Source: CAD feature listing. Evaluate the final solid. Frame: model axes, mm. A direction names the side the tool comes from. Round coordinates to 2 decimals unless told otherwise and drop trailing zeros. Answer in a Markdown table with one row per item. Add a question column.
Item 1: Mould query, pull axis Y, two halves, no side actions, for faces 1 (the face through (-2, 212.5, 7)), 2 (the face through (16, 158, 6)), 3 (the face through (-161, -3, 7)). Classes: released by +Y, released by -Y, zero draft, split by the parting line, or undercut.
Item 2: Set-up query: faces 4 (the face through (134, -112, 8)), 5 (the face through (-2, 3, 0)). Return all of +Z, -Z, +X, -X, +Y, -Y with unobstructed straight access to the full face (end or side cutting, diameter ignored); none if empty.
Item 3: Material intervals for probe 1 along Y at (x, z) = (-14.3, 1.5); probe 2 along Y at (x, z) = (152.5, 6.5); probe 3 along X at (y, z) = (144.5, 4), sorted ascending.
Item 4: Contact query for flat-ended pins moving along their axis: pin 1 (3.5 mm diameter, centred on x = 96.5, y = 109.5, fed in from +Z); pin 2 (3 mm diameter, centred on x = -94.5, y = -111.5, fed in from +Z). Output: stop coordinate, or through.
from build123d import *

# Parameters (mm, degrees)
SZKIC1_W                       = 322
SZKIC1_H                       = 425
DODANIE_WYCI_GNI_CIE1_DEPTH    = 15
SZKIC2_R                       = 3
WYTNIJ_WYCI_GNI_CIE1_DEPTH     = 15
SZKIC3_R                       = 5
WYTNIJ_WYCI_GNI_CIE2_DEPTH     = 7
SZYK_LINIOWY1_COUNT            = 2
SZYK_LINIOWY1_PITCH            = 35
SZYK_LINIOWY1_COUNT_DIR2       = 2
SZYK_LINIOWY1_PITCH_DIR2       = 35
SZYK_LINIOWY2_COUNT            = 2
SZYK_LINIOWY2_PITCH            = 228
SZYK_LINIOWY2_COUNT_DIR2       = 2
SZYK_LINIOWY2_PITCH_DIR2       = 254
SZYK_LINIOWY2_COPY_1_SKETCH_R  = 3
SZYK_LINIOWY2_COPY_1_DEPTH     = 15
SZYK_LINIOWY2_COPY_2_SKETCH_R  = 3
SZYK_LINIOWY2_COPY_2_DEPTH     = 15
SZYK_LINIOWY2_COPY_3_SKETCH_R  = 3
SZYK_LINIOWY2_COPY_3_DEPTH     = 15
SZYK_LINIOWY2_COPY_4_SKETCH_R  = 3
SZYK_LINIOWY2_COPY_4_DEPTH     = 15
SZYK_LINIOWY2_COPY_5_SKETCH_R  = 3
SZYK_LINIOWY2_COPY_5_DEPTH     = 15
SZYK_LINIOWY2_COPY_6_SKETCH_R  = 3
SZYK_LINIOWY2_COPY_6_DEPTH     = 15
SZYK_LINIOWY2_COPY_7_SKETCH_R  = 3
SZYK_LINIOWY2_COPY_7_DEPTH     = 15
SZYK_LINIOWY2_COPY_8_SKETCH_R  = 3
SZYK_LINIOWY2_COPY_8_DEPTH     = 15
SZYK_LINIOWY2_COPY_9_SKETCH_R  = 3
SZYK_LINIOWY2_COPY_9_DEPTH     = 15
SZYK_LINIOWY2_COPY_10_SKETCH_R = 5
SZYK_LINIOWY2_COPY_10_DEPTH    = 7
SZYK_LINIOWY2_COPY_11_SKETCH_R = 5
SZYK_LINIOWY2_COPY_11_DEPTH    = 7
SZYK_LINIOWY2_COPY_12_SKETCH_R = 5
SZYK_LINIOWY2_COPY_12_DEPTH    = 7
SZYK_LINIOWY2_COPY_13_SKETCH_R = 5
SZYK_LINIOWY2_COPY_13_DEPTH    = 7
SZYK_LINIOWY2_COPY_14_SKETCH_R = 5
SZYK_LINIOWY2_COPY_14_DEPTH    = 7
SZYK_LINIOWY2_COPY_15_SKETCH_R = 5
SZYK_LINIOWY2_COPY_15_DEPTH    = 7
SZYK_LINIOWY2_COPY_16_SKETCH_R = 5
SZYK_LINIOWY2_COPY_16_DEPTH    = 7
SZYK_LINIOWY2_COPY_17_SKETCH_R = 5
SZYK_LINIOWY2_COPY_17_DEPTH    = 7
SZYK_LINIOWY2_COPY_18_SKETCH_R = 5
SZYK_LINIOWY2_COPY_18_DEPTH    = 7
SZKIC6_R                       = 4
WYTNIJ_WYCI_GNI_CIE3_DEPTH     = 20
SZKIC7_R                       = 4
WYTNIJ_WYCI_GNI_CIE4_DEPTH     = 20
SZKIC10_R                      = 4
WYTNIJ_WYCI_GNI_CIE5_DEPTH     = 21
SZKIC11_R                      = 4
WYTNIJ_WYCI_GNI_CIE6_DEPTH     = 21
SZKIC12_R                      = 3.999999999
WYTNIJ_WYCI_GNI_CIE7_DEPTH     = 15
SZKIC13_R                      = 6.499999999
WYTNIJ_WYCI_GNI_CIE8_DEPTH     = 9
SZKIC14_R                      = 4
WYTNIJ_WYCI_GNI_CIE9_DEPTH     = 15
SZYK_LINIOWY3_COUNT            = 4
SZYK_LINIOWY3_PITCH            = 133


with BuildPart() as part:
    # Szkic1 → Dodanie-wyciągnięcie1 (new body)
    with BuildSketch(Plane.XY):
        Rectangle(SZKIC1_W, SZKIC1_H)
    extrude(amount=DODANIE_WYCI_GNI_CIE1_DEPTH)

    # Szkic2 → Wytnij-wyciągnięcie1 (cut)
    with BuildSketch(Plane.XY.offset(15)):
        with Locations((-131.5, 144.5)):
            Circle(SZKIC2_R)
    wytnij_wyci_gni_cie1 = extrude(amount=-WYTNIJ_WYCI_GNI_CIE1_DEPTH, mode=Mode.SUBTRACT)

    # Szkic3 → Wytnij-wyciągnięcie2 (cut)
    with BuildSketch(Plane.XY.offset(15)):
        with Locations((-131.5, 144.5)):
            Circle(SZKIC3_R)
    wytnij_wyci_gni_cie2 = extrude(amount=-WYTNIJ_WYCI_GNI_CIE2_DEPTH, mode=Mode.SUBTRACT)

    # Szyk liniowy1: Wytnij-wyciągnięcie1, Wytnij-wyci_gni_cie2 2 × 2
    with Locations(*[(i * SZYK_LINIOWY1_PITCH, -j * SZYK_LINIOWY1_PITCH_DIR2, 0) for i in range(SZYK_LINIOWY1_COUNT) for j in range(SZYK_LINIOWY1_COUNT_DIR2) if (i, j) != (0, 0)]):
        add(wytnij_wyci_gni_cie1, mode=Mode.SUBTRACT)
        add(wytnij_wyci_gni_cie2, mode=Mode.SUBTRACT)

    # Szyk liniowy2: Wytnij-wyciągnięcie1, Wytnij-wyci_gni_cie2 2 × 2
    with Locations(*[(i * SZYK_LINIOWY2_PITCH, -j * SZYK_LINIOWY2_PITCH_DIR2, 0) for i in range(SZYK_LINIOWY2_COUNT) for j in range(SZYK_LINIOWY2_COUNT_DIR2) if (i, j) != (0, 0)]):
        add(wytnij_wyci_gni_cie1, mode=Mode.SUBTRACT)
        add(wytnij_wyci_gni_cie2, mode=Mode.SUBTRACT)

    # Szyk liniowy2 copy 1 sketch → Szyk liniowy2 copy 1 (cut)
    with BuildSketch(Plane(origin=(0, -289, 15), x_dir=(1, 0, 0), z_dir=(0, 0, 1))):
        with Locations((-131.5, 144.5)):
            Circle(SZYK_LINIOWY2_COPY_1_SKETCH_R)
    extrude(amount=-SZYK_LINIOWY2_COPY_1_DEPTH, mode=Mode.SUBTRACT)

    # Szyk liniowy2 copy 2 sketch → Szyk liniowy2 copy 2 (cut)
    with BuildSketch(Plane(origin=(228, -35, 15), x_dir=(1, 0, 0), z_dir=(0, 0, 1))):
        with Locations((-131.5, 144.5)):
            Circle(SZYK_LINIOWY2_COPY_2_SKETCH_R)
    extrude(amount=-SZYK_LINIOWY2_COPY_2_DEPTH, mode=Mode.SUBTRACT)

    # Szyk liniowy2 copy 3 sketch → Szyk liniowy2 copy 3 (cut)
    with BuildSketch(Plane(origin=(228, -289, 15), x_dir=(1, 0, 0), z_dir=(0, 0, 1))):
        with Locations((-131.5, 144.5)):
            Circle(SZYK_LINIOWY2_COPY_3_SKETCH_R)
    extrude(amount=-SZYK_LINIOWY2_COPY_3_DEPTH, mode=Mode.SUBTRACT)

    # Szyk liniowy2 copy 4 sketch → Szyk liniowy2 copy 4 (cut)
    with BuildSketch(Plane(origin=(35, -254, 15), x_dir=(1, 0, 0), z_dir=(0, 0, 1))):
        with Locations((-131.5, 144.5)):
            Circle(SZYK_LINIOWY2_COPY_4_SKETCH_R)
    extrude(amount=-SZYK_LINIOWY2_COPY_4_DEPTH, mode=Mode.SUBTRACT)

    # Szyk liniowy2 copy 5 sketch → Szyk liniowy2 copy 5 (cut)
    with BuildSketch(Plane(origin=(263, 0, 15), x_dir=(1, 0, 0), z_dir=(0, 0, 1))):
        with Locations((-131.5, 144.5)):
            Circle(SZYK_LINIOWY2_COPY_5_SKETCH_R)
    extrude(amount=-SZYK_LINIOWY2_COPY_5_DEPTH, mode=Mode.SUBTRACT)

    # Szyk liniowy2 copy 6 sketch → Szyk liniowy2 copy 6 (cut)
    with BuildSketch(Plane(origin=(263, -254, 15), x_dir=(1, 0, 0), z_dir=(0, 0, 1))):
        with Locations((-131.5, 144.5)):
            Circle(SZYK_LINIOWY2_COPY_6_SKETCH_R)
    extrude(amount=-SZYK_LINIOWY2_COPY_6_DEPTH, mode=Mode.SUBTRACT)

    # Szyk liniowy2 copy 7 sketch → Szyk liniowy2 copy 7 (cut)
    with BuildSketch(Plane(origin=(35, -289, 15), x_dir=(1, 0, 0), z_dir=(0, 0, 1))):
        with Locations((-131.5, 144.5)):
            Circle(SZYK_LINIOWY2_COPY_7_SKETCH_R)
    extrude(amount=-SZYK_LINIOWY2_COPY_7_DEPTH, mode=Mode.SUBTRACT)

    # Szyk liniowy2 copy 8 sketch → Szyk liniowy2 copy 8 (cut)
    with BuildSketch(Plane(origin=(263, -35, 15), x_dir=(1, 0, 0), z_dir=(0, 0, 1))):
        with Locations((-131.5, 144.5)):
            Circle(SZYK_LINIOWY2_COPY_8_SKETCH_R)
    extrude(amount=-SZYK_LINIOWY2_COPY_8_DEPTH, mode=Mode.SUBTRACT)

    # Szyk liniowy2 copy 9 sketch → Szyk liniowy2 copy 9 (cut)
    with BuildSketch(Plane(origin=(263, -289, 15), x_dir=(1, 0, 0), z_dir=(0, 0, 1))):
        with Locations((-131.5, 144.5)):
            Circle(SZYK_LINIOWY2_COPY_9_SKETCH_R)
    extrude(amount=-SZYK_LINIOWY2_COPY_9_DEPTH, mode=Mode.SUBTRACT)

    # Szyk liniowy2 copy 10 sketch → Szyk liniowy2 copy 10 (cut)
    with BuildSketch(Plane(origin=(0, -289, 15), x_dir=(1, 0, 0), z_dir=(0, 0, 1))):
        with Locations((-131.5, 144.5)):
            Circle(SZYK_LINIOWY2_COPY_10_SKETCH_R)
    extrude(amount=-SZYK_LINIOWY2_COPY_10_DEPTH, mode=Mode.SUBTRACT)

    # Szyk liniowy2 copy 11 sketch → Szyk liniowy2 copy 11 (cut)
    with BuildSketch(Plane(origin=(228, -35, 15), x_dir=(1, 0, 0), z_dir=(0, 0, 1))):
        with Locations((-131.5, 144.5)):
            Circle(SZYK_LINIOWY2_COPY_11_SKETCH_R)
    extrude(amount=-SZYK_LINIOWY2_COPY_11_DEPTH, mode=Mode.SUBTRACT)

    # Szyk liniowy2 copy 12 sketch → Szyk liniowy2 copy 12 (cut)
    with BuildSketch(Plane(origin=(228, -289, 15), x_dir=(1, 0, 0), z_dir=(0, 0, 1))):
        with Locations((-131.5, 144.5)):
            Circle(SZYK_LINIOWY2_COPY_12_SKETCH_R)
    extrude(amount=-SZYK_LINIOWY2_COPY_12_DEPTH, mode=Mode.SUBTRACT)

    # Szyk liniowy2 copy 13 sketch → Szyk liniowy2 copy 13 (cut)
    with BuildSketch(Plane(origin=(35, -254, 15), x_dir=(1, 0, 0), z_dir=(0, 0, 1))):
        with Locations((-131.5, 144.5)):
            Circle(SZYK_LINIOWY2_COPY_13_SKETCH_R)
    extrude(amount=-SZYK_LINIOWY2_COPY_13_DEPTH, mode=Mode.SUBTRACT)

    # Szyk liniowy2 copy 14 sketch → Szyk liniowy2 copy 14 (cut)
    with BuildSketch(Plane(origin=(263, 0, 15), x_dir=(1, 0, 0), z_dir=(0, 0, 1))):
        with Locations((-131.5, 144.5)):
            Circle(SZYK_LINIOWY2_COPY_14_SKETCH_R)
    extrude(amount=-SZYK_LINIOWY2_COPY_14_DEPTH, mode=Mode.SUBTRACT)

    # Szyk liniowy2 copy 15 sketch → Szyk liniowy2 copy 15 (cut)
    with BuildSketch(Plane(origin=(263, -254, 15), x_dir=(1, 0, 0), z_dir=(0, 0, 1))):
        with Locations((-131.5, 144.5)):
            Circle(SZYK_LINIOWY2_COPY_15_SKETCH_R)
    extrude(amount=-SZYK_LINIOWY2_COPY_15_DEPTH, mode=Mode.SUBTRACT)

    # Szyk liniowy2 copy 16 sketch → Szyk liniowy2 copy 16 (cut)
    with BuildSketch(Plane(origin=(35, -289, 15), x_dir=(1, 0, 0), z_dir=(0, 0, 1))):
        with Locations((-131.5, 144.5)):
            Circle(SZYK_LINIOWY2_COPY_16_SKETCH_R)
    extrude(amount=-SZYK_LINIOWY2_COPY_16_DEPTH, mode=Mode.SUBTRACT)

    # Szyk liniowy2 copy 17 sketch → Szyk liniowy2 copy 17 (cut)
    with BuildSketch(Plane(origin=(263, -35, 15), x_dir=(1, 0, 0), z_dir=(0, 0, 1))):
        with Locations((-131.5, 144.5)):
            Circle(SZYK_LINIOWY2_COPY_17_SKETCH_R)
    extrude(amount=-SZYK_LINIOWY2_COPY_17_DEPTH, mode=Mode.SUBTRACT)

    # Szyk liniowy2 copy 18 sketch → Szyk liniowy2 copy 18 (cut)
    with BuildSketch(Plane(origin=(263, -289, 15), x_dir=(1, 0, 0), z_dir=(0, 0, 1))):
        with Locations((-131.5, 144.5)):
            Circle(SZYK_LINIOWY2_COPY_18_SKETCH_R)
    extrude(amount=-SZYK_LINIOWY2_COPY_18_DEPTH, mode=Mode.SUBTRACT)

    # Szkic6 → Wytnij-wyciągnięcie3 (cut)
    with BuildSketch(Plane.XY.offset(15)):
        with Locations((-152.5, 199.5)):
            Circle(SZKIC6_R)
        with Locations((-75.5, 199.5)):
            Circle(SZKIC6_R)
    extrude(amount=-WYTNIJ_WYCI_GNI_CIE3_DEPTH, mode=Mode.SUBTRACT)

    # Szkic7 → Wytnij-wyciągnięcie4 (cut)
    with BuildSketch(Plane.XY.offset(15)):
        with Locations((-152.5, -204)):
            Circle(SZKIC7_R)
        with Locations((-152.5, -179)):
            Circle(SZKIC7_R)
        with Locations((-75.5, -204)):
            Circle(SZKIC7_R)
        with Locations((-75.5, -179)):
            Circle(SZKIC7_R)
    extrude(amount=-WYTNIJ_WYCI_GNI_CIE4_DEPTH, mode=Mode.SUBTRACT)

    # Szkic10 → Wytnij-wyciągnięcie5 (cut)
    with BuildSketch(Plane.XY.offset(15)):
        with Locations((75.5, 199.5)):
            Circle(SZKIC10_R)
        with Locations((152.5, 199.5)):
            Circle(SZKIC10_R)
    extrude(amount=-WYTNIJ_WYCI_GNI_CIE5_DEPTH, mode=Mode.SUBTRACT)

    # Szkic11 → Wytnij-wyciągnięcie6 (cut)
    with BuildSketch(Plane.XY.offset(15)):
        with Locations((152.5, -179)):
            Circle(SZKIC11_R)
        with Locations((152.5, -204)):
            Circle(SZKIC11_R)
        with Locations((75.5, -204)):
            Circle(SZKIC11_R)
        with Locations((75.5, -179)):
            Circle(SZKIC11_R)
    extrude(amount=-WYTNIJ_WYCI_GNI_CIE6_DEPTH, mode=Mode.SUBTRACT)

    # Szkic12 → Wytnij-wyciągnięcie7 (cut)
    with BuildSketch(Plane.XY.offset(15)):
        with Locations((-14.3, 205.5)):
            Circle(SZKIC12_R)
        with Locations((11.7, 205.5)):
            Circle(SZKIC12_R)
        with Locations((-14.3, 157.5)):
            Circle(SZKIC12_R)
        with Locations((11.7, 157.5)):
            Circle(SZKIC12_R)
    extrude(amount=-WYTNIJ_WYCI_GNI_CIE7_DEPTH, mode=Mode.SUBTRACT)

    # Szkic13 → Wytnij-wyciągnięcie8 (cut)
    with BuildSketch(Plane.XY.offset(15)):
        with Locations((-14.3, 205.5)):
            Circle(SZKIC13_R)
        with Locations((11.7, 205.5)):
            Circle(SZKIC13_R)
        with Locations((11.7, 157.5)):
            Circle(SZKIC13_R)
        with Locations((-14.3, 157.5)):
            Circle(SZKIC13_R)
    extrude(amount=-WYTNIJ_WYCI_GNI_CIE8_DEPTH, mode=Mode.SUBTRACT)

    # Szkic14 → Wytnij-wyciągnięcie9 (cut)
    with BuildSketch(Plane.XY.offset(15)):
        with Locations((-54, 199.5)):
            Circle(SZKIC14_R)
        with Locations((54, 199.5)):
            Circle(SZKIC14_R)
    wytnij_wyci_gni_cie9 = extrude(amount=-WYTNIJ_WYCI_GNI_CIE9_DEPTH, mode=Mode.SUBTRACT)

    # Szyk liniowy3: Wytnij-wyciągnięcie9 ×4
    with Locations(*[(0, -i * SZYK_LINIOWY3_PITCH, 0) for i in range(1, SZYK_LINIOWY3_COUNT)]):
        add(wytnij_wyci_gni_cie9, mode=Mode.SUBTRACT)


solid = part.part
Results below:
| question | item | result |
|---|---|---|
| 1 | face 1 | released by +Y |
| 1 | face 2 | undercut |
| 1 | face 3 | zero draft |
| 2 | face 4 | +Z |
| 2 | face 5 | -Z, +X, -X, +Y, -Y |
| 3 | probe 1 | -212.5 to 153.5, 161.5 to 201.5, 209.5 to 212.5 |
| 3 | probe 2 | -212.5 to -208, -200 to -183, -175 to 195.5, 203.5 to 212.5 |
| 3 | probe 3 | -161 to -134.5, -128.5 to -99.5, -93.5 to 93.5, 99.5 to 128.5, 134.5 to 161 |
| 4 | pin 1 | through |
| 4 | pin 2 | z = 8 |
